Autodesk Inventor part; units mm, degrees
ref_plane "YZ Plane" through (0, 0, 0) normal (1, 0, 0) x (0, 1, 0)
ref_plane "XZ Plane" through (0, 0, 0) normal (0, 1, 0) x (-1, 0, 0)
ref_plane "XY Plane" through (0, 0, 0) normal (0, 0, 1) x (1, 0, 0)
sketch "Boceto1" plane through (0, 0, 0) normal (0, 1, 0) x (-1, 0, 0)
  line L0 (-9.85, 9.85) -> (9.85, 9.85)
  line L1 (9.85, 9.85) -> (9.85, -9.85)
  line L2 (9.85, -9.85) -> (-9.85, -9.85)
  line L3 (-9.85, -9.85) -> (-9.85, 9.85)
  line L4 (-9.85, 9.85) -> (9.85, -9.85) construction
  line L5 (9.85, 9.85) -> (-9.85, -9.85) construction
  point P0 (0, 0)
  dimension "d0" = 19.7
  dimension "d1" = 19.7
extrude "Extrusión1" add sketch "Boceto1" along normal blind 7
sketch "Boceto2" plane through (0, 7, 0) normal (0, 1, 0) x (1, 0, 0)
  line L0 (-9.85, -9.85) -> (9.85, -9.85)
  line L1 (9.85, -9.85) -> (16.45, -9.85)
  line L2 (16.45, -9.85) -> (16.45, 9.85)
  line L3 (16.45, 9.85) -> (9.85, 9.85)
  line L4 (9.85, 9.85) -> (9.85, -9.85)
  line L5 (9.85, 9.85) -> (-9.85, 9.85)
  point P0 (0, 0)
  dimension "d4" = 6.6
extrude "Extrusión2" add sketch "Boceto2" against normal blind 30
sketch "Boceto3" plane through (16.45, 7, 9.85) normal (1, 0, 0) x (0, 0, -1)
  circle A0 centre (9.435, -20) radius 2.7
  line L0 (19.7, -30) -> (0, -30)
  point P0 (9.85, -7)
  dimension "d7" = 5.4
  dimension "d8" = 10
extrude "Extrusión3" cut sketch "Boceto3" against normal blind 20
sketch "Boceto4" plane through (16.45, 7, 9.85) normal (1, 0, 0) x (0, 0, -1)
  circle A0 centre (9.435, -20) radius 2.7
  circle A1 centre (9.435, -20) radius 4.65
  point P0 (9.85, -7)
  dimension "d11" = 9.3
extrude "Extrusión4" cut sketch "Boceto4" against normal blind 2 contours A0 | A1
sketch "Boceto5" plane through (0, 7, 0) normal (0, 1, 0) x (1, 0, 0)
  circle A0 centre (0, 0) radius 2.7
  dimension "d14" = 5.4
extrude "Extrusión5" cut sketch "Boceto5" against normal through all
sketch "Boceto6" plane through (0, 0, 0) normal (0, -1, 0) x (1, 0, 0)
  circle A0 centre (0, 0) radius 4.05
  line L0 (0, 4.6765) -> (4.05, 2.3383)
  line L1 (4.05, 2.3383) -> (4.05, -2.3383)
  line L2 (4.05, -2.3383) -> (0, -4.6765)
  line L3 (0, -4.6765) -> (-4.05, -2.3383)
  line L4 (-4.05, -2.3383) -> (-4.05, 2.3383)
  line L5 (-4.05, 2.3383) -> (0, 4.6765)
  dimension "d17" = 8.1
extrude "Extrusión6" cut sketch "Boceto6" against normal blind 4.1
fillet "Empalme1" radius 3 3 edges at (16.45, 7, 0) (13.15, -23, 9.85) (13.15, -23, -9.85)
sketch "Boceto8" plane through (0, 0, 0) normal (0, -1, 0) x (1, 0, 0)
  line L0 (10.15, -10.15) -> (-10.15, -10.15)
  line L1 (-10.15, -10.15) -> (-10.15, 10.15)
  line L2 (-10.15, 10.15) -> (10.15, 10.15)
  line L3 (10.15, 10.15) -> (10.15, -10.15)
  line L4 (10.15, -10.15) -> (-10.15, 10.15) construction
  line L5 (-10.15, -10.15) -> (10.15, 10.15) construction
  point P0 (0, 0)
  dimension "d21" = 20.3
  dimension "d22" = 20.3
extrude "Extrusión7" cut sketch "Boceto8" along normal through all
fillet "Empalme2" radius 3 2 edges at (-9.85, 3.5, 9.85) (-9.85, 3.5, -9.85)
properties part number "soportetuerca"
Model file for the job. Use its own axes, mm. A direction names the side the tool comes from. Round coordinates to 2 decimals unless told otherwise and drop trailing zeros. Loops run counter-clockwise (first coordinate to the right, second up) from the corner with the lowest first, then second, coordinate; pieces in that order, holes last. Notation, with made-up numbers: M 68.5,-37 L 85.5,-37 A31 cw 85.5,-1 Z; hole C 62.25,48 d8. An arc over 180 degrees is marked long. Put each result on its own line as item: value. Start each with the question number.
Item 1: Cut at A-A (y = -13). List the corners of the cut face in (x, z) (3 decimals).
Item 2: Cut at D-D (x = 14). List the corners of the cut face in (y, z) (3 decimals).
Item 3: Drill centre lines: line 1 along X through (y, z) = (1.25, -1); line 2 along Z through (x, y) = (0, 5.1); line 3 along Y through (x, z) = (8.5, -2.25). Where is each one in solid material? Low to high.
Item 4: Mould opens along Y. For faces 1 (the face through (14.45, -15, -2)), 2 (the face through (-3, 4.1, 0)), 3 (the face through (12, -1, -9.85)) say: released by +Y, released by -Y, zero draft, split by the parting line, or undercut.
Item 5: 3-axis set-ups, long thin cutter, end or side, ignore diameter. For faces 4 (the face through (15.46, -17.54, 1.42)), 5 (the face through (-4.05, 2, 0)), 6 (the face through (0, 0, 5)): which of +Z, -Z, +X, -X, +Y, -Y reach the whole face in a straight line?
Item 6: Cut at B-B (z = -1.5). List the corners of the cut face in (x, y) (3 decimals).
Item 7: Drop flat-ended pins along their axis: P1, Ø2, axis at y = -16, z = 1, coming from the +X side; P2, Ø2, axis at x = -6.5, z = -4.5, coming from the -Y side; P3, Ø5.5, axis at y = -13, z = 0.415, coming from the -X side. Give the stop position or say it passes through.
Answer block:
1. outline: M 10.15,-9.85 L 16.45,-9.85 L 16.45,-4.235 L 14.45,-4.235 L 14.45,-2.285 L 10.15,-2.285 Z; M 10.15,3.115 L 14.45,3.115 L 14.45,5.065 L 16.45,5.065 L 16.45,9.85 L 10.15,9.85 Z
2. outline: M -23,-6.85 A3 ccw -20,-9.85 L 6.949,-9.85 L 6.949,9.85 L -20,9.85 A3 ccw -23,6.85 Z; hole C -13,0.415 d5.4
3. line 1: -9.85 to -4.05, 4.05 to 16.45
3. line 2: -9.85 to -2.7, 2.7 to 9.85
3. line 3: 0 to 7
4. face 1: undercut
4. face 2: released by -Y
4. face 3: zero draft
5. face 4: +X
5. face 5: -Y
5. face 6: +Z, -Z, -X, -Y
6. outline: M -9.85,0 L -4.05,0 L -4.05,4.1 L -2.245,4.1 L -2.245,7 L -9.85,7 Z; M 2.245,4.1 L 4.05,4.1 L 4.05,0 L 10.15,0 L 10.15,-11.097 L 14.45,-11.097 L 14.45,-8.763 L 16.45,-8.763 L 16.45,4 A3 ccw 13.45,7 L 2.245,7 Z; M 10.15,-23 L 16.45,-23 L 16.45,-17.237 L 14.45,-17.237 L 14.45,-14.903 L 10.15,-14.903 Z
7. P1: x = 14.45
7. P2: y = 0
7. P3: x = 10.15
